from build123d import *

# Parameters (mm, degrees)
BOSS_EXTRUDE1_DEPTH = 0.8
FILLET1_R           = 2


with BuildPart() as part:
    # Sketch1 → Boss-Extrude1 (new body)
    with BuildSketch(Plane.XY):
        with BuildLine():
            Line((14.5, 0), (48.1, 0))
            Line((48.1, 0), (48.1, 70))
            Line((48.1, 70), (48.9, 70))
            Line((48.9, 70), (48.9, 0))
            Line((48.9, 0), (82.5, 0))
            ThreePointArc((82.5, 0), (92.968719423, 7.187289944), (97, 19.228884523))
            Line((97, 19.228884523), (97, 124))
            Line((97, 124), (89, 132))
            Line((89, 132), (84.5, 132))
            Line((84.5, 132), (84.5, 136))
            Line((84.5, 136), (45.939865431, 136))
            Line((45.939865431, 136), (12.5, 136))
            Line((12.5, 136), (12.5, 132))
            Line((12.5, 132), (8, 132))
            Line((8, 132), (0, 124))
            Line((0, 124), (0, 19.228884523))
            ThreePointArc((0, 19.228884523), (4.031280577, 7.187289944), (14.5, 0))
        make_face()
    extrude(amount=BOSS_EXTRUDE1_DEPTH)

    # Fillet1
    fillet1_edges = [part.edges().sort_by_distance(p)[0] for p in [
        (89, 132, 0.4),
        (97, 124, 0.4),
        (0, 124, 0.4),
        (8, 132, 0.4),
    ]]
    fillet(fillet1_edges, radius=FILLET1_R)


solid = part.part
Geometry: final body of the model. Coordinates: model frame, mm. Round coordinates to 2 decimals unless told otherwise and drop trailing zeros. Loops run counter-clockwise (first coordinate to the right, second up) from the corner with the lowest first, then second, coordinate; pieces in that order, holes last. Notation, with made-up numbers: M -36.75,81.5 L -5.75,81.5 A18 cw -5.75,111.5 Z; hole C 7.25,-40 d11. An arc over 180 degrees is marked long. Put each result on its own line as item: value. Start each with the question number.
(1) Section query C-C (x = 10.5). Return loops of the section in (y, z).
(2) Section query B-B (y = 14). Return loops of the section in (x, z), then the cut area to 3 significant figures.
(3) Section query A-A (z = 0.2). Return loops of the section in (x, y), then the cut area to 3 significant figures.
(4) Material intervals for line 1 along X through (y, z) = (53, 0.55); line 2 along Y through (x, z) = (5.5, 0.15); line 3 along Y through (x, z) = (88.5, 0.25), sorted ascending. Write a range as [from, to].
Findings below:
1. outline: M 1.63,0 L 132,0 L 132,0.8 L 1.63,0.8 Z
2. outline: M 0.7,0 L 48.1,0 L 48.1,0.8 L 0.7,0.8 Z; M 48.9,0 L 96.3,0 L 96.3,0.8 L 48.9,0.8 Z
2. area: 75.8 mm2
3. outline: M 0,19.23 A20 ccw 14.5,0 L 48.1,0 L 48.1,70 L 48.9,70 L 48.9,0 L 82.5,0 A20 ccw 97,19.23 L 97,123.17 A2 ccw 96.41,124.59 L 89.59,131.41 A2 ccw 88.17,132 L 84.5,132 L 84.5,136 L 12.5,136 L 12.5,132 L 8.83,132 A2 ccw 7.41,131.41 L 0.59,124.59 A2 ccw 0,123.17 Z
3. area: 12,800 mm2
4. line 1: x = [0, 48.1], [48.9, 97]
4. line 2: y = [5.45, 129.5]
4. line 3: y = [2.87, 131.97]
